Part print with two shaded views. Sizes in mm from the minimum x, y, z corner. A direction names the side the tool comes from. Give positions to 0.01 mm unless a question says otherwise; leave off trailing zeros. Order: outer loops, then holes, each group sorted by start corner. A loop starts at its lowest first (then second) coordinate and runs counter-clockwise, first axis right, second up. Notation, with made-up numbers: M -17.5,45.5 L 9.5,45.5 A26 ccw 9.5,76.5 Z; hole C 68.25,14.5 d10. An arc over 180 degrees is marked long. Return JSON: item names as keys, results as strings. Group by question number.
1. Pin check, flat tips, straight feed: pin 1 (5 mm diameter, centred on x = 5.5, y = 14, fed in from +Z); pin 2 (8 mm diameter, centred on x = 6.5, y = 29.5, fed in from +Z); pin 3 (1 mm diameter, centred on y = 14.5, z = 23, fed in from -X). Stop position of each tip, or through.
2. Slice it at C-C on x = 10.75. List the corners of the cut face in (y, z) (3 decimals), then the cut area to 3 significant figures.
3. 3-axis set-ups, long thin cutter, end or side, ignore diameter. For the marked faces 1, 2 and 3: which of +Z, -Z, +X, -X, +Y, -Y reach the whole face in a straight line?
4. Two-plate mould, pull along Y, no slides. Class the marked faces 4, 5 and 6: released by +Y, released by -Y, zero draft, split by the parting line, or undercut.
5. Wall check: probe 1 along Y at (x, z) = (2, 20) (3 decimals); probe 2 along Z at (x, y) = (12.5, 24). Give the ranges that are in metal, low to high. Write a range as [from, to].
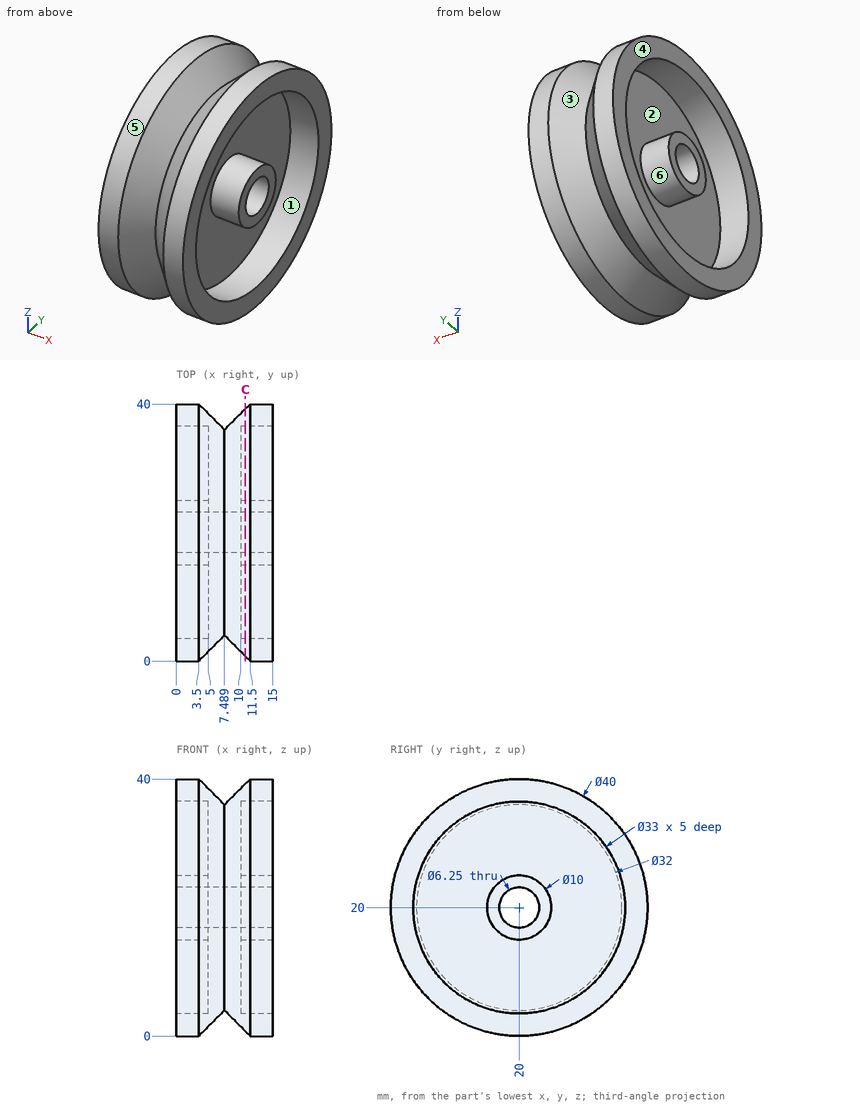
Result:
{
 "1": {"pin 1": "stops at z = 39.49", "pin 2": "stops at z = 38.79", "pin 3": "stops at x = 5"},
 "2": {"outline": "C 20,20 d38.504; C 20,20 d10; hole C 20,20 d33; hole C 20,20 d6.25", "area": "357 mm2"},
 "3": {"face 1": "+X", "face 2": "-X", "face 3": "none"},
 "4": {"face 4": "zero draft", "face 5": "split by the parting line", "face 6": "undercut"},
 "5": {"probe 1": "y = [0, 3.5], [15, 16.875], [23.125, 25], [36.5, 40]", "probe 2": "z = [0.4, 3.99], [17, 23], [36.01, 39.6]"}
}
